The listing builds one solid part. Answer for the finished solid, in the listing's coordinates (mm). Face numbers are marked on the shaded views. A direction names the side the tool comes from. Give positions to 0.01 mm unless a question says otherwise; leave off trailing zeros. Write each loop counter-clockwise with the first axis right and the second up, starting at its lowest first coordinate (ties: lowest second). Pieces come first, ordered by that corner, then holes. Notation, with made-up numbers: M 34.25,2.25 L 89.25,2.25 A21 ccw 89.25,37.25 Z; hole C 57,-31 d10. An arc over 180 degrees is marked long. Return JSON: item names as keys, results as strings.
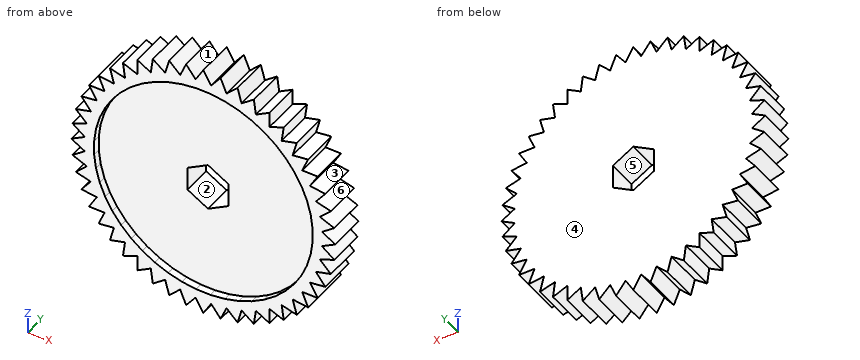
from build123d import *

# Parameters (mm, degrees)
SKETCH1_R           = 19.05
BOSS_EXTRUDE1_DEPTH = 5.08
BOSS_EXTRUDE3_DEPTH = 6.35
CIRPATTERN1_COUNT   = 48
CUT_EXTRUDE1_DEPTH  = 33.725610766


with BuildPart() as part:
    # Sketch1 → Boss-Extrude1 (new body)
    with BuildSketch(Plane(origin=(0, 0, 0), x_dir=(1, 0, 0), z_dir=(0, 1, 0))):
        with Locations(Location((0, 0, 0), (0, 0, 270))):
            Circle(SKETCH1_R)
    extrude(amount=BOSS_EXTRUDE1_DEPTH)

    # Sketch3 → Boss-Extrude3 (add)
    with BuildSketch(Plane(origin=(0, 5.08, 0), x_dir=(1, 0, 0), z_dir=(0, 1, 0))):
        Polygon((0, 22.86), (2.278670365, 18.913227154), (-2.278670365, 18.913227154), align=None)
    boss_extrude3 = extrude(amount=-BOSS_EXTRUDE3_DEPTH)

    # CirPattern1: Boss-Extrude3 ×48 about axis
    cirpattern1_axis = Axis((0, 0, 0), (0, 1, 0))
    for i in range(1, CIRPATTERN1_COUNT):
        add(boss_extrude3.rotate(cirpattern1_axis, i * 360 / CIRPATTERN1_COUNT))

    # Sketch6 → Cut-Extrude1 (cut, through all)
    with BuildSketch(Plane.XZ):
        Polygon((0, -4.106115114), (3.556, -2.053057557), (3.556, 2.053057557), (0, 4.106115114), (-3.556, 2.053057557), (-3.556, -2.053057557), align=None)
    extrude(amount=-CUT_EXTRUDE1_DEPTH, mode=Mode.SUBTRACT)


solid = part.part
Item 1: Which of the six approach directions +Z, -Z, +X, -X, +Y, -Y give full straight-line access (tool end or side, diameter ignored) to the marked faces 1, 2 and 3?
Geometry results:
{"face 1": "+Z, +Y, -Y", "face 2": "+Y, -Y", "face 3": "+X, +Y, -Y"}
Item 2: A cutting plane is placed at A-A, the plane z = -5. Write down the section's boundary in (x, y).
Geometry results:
{"outline": "M -21.16,-1.27 L -18.24,-1.27 L -18.24,0 L 18.24,0 L 18.24,-1.27 L 21.16,-1.27 L 21.16,5.08 L -21.16,5.08 Z"}
Item 3: A cutting plane is placed at B-B, the plane x = 10. Write down the section's boundary in (y, z).
Geometry results:
{"outline": "M -1.27,-18.97 L 5.08,-18.97 L 5.08,18.97 L -1.27,18.97 L -1.27,16.07 L 0,16.07 L 0,-16.07 L -1.27,-16.07 Z"}
Item 4: Determine the mould class of the marked faces 4, 5 and 6 for opening direction X: +X half, -X half, draft (parallel to the pull), parting line (faces both ways), or undercut.
Geometry results:
{"face 4": "draft", "face 5": "undercut", "face 6": "+X half"}
Item 5: Given pin 1 Ø3 at (y, z) = (3.5, -18) entering from +X; pin 2 Ø1.3 at (x, y) = (-18, 1.5) entering from -Z; pin 3 Ø0.8 at (y, z) = (3, 18.5) entering from -X, each flat-ended and moving along its own axis, determine where each tip first touches the part or whether it passes through.
Geometry results:
{"pin 1": "stops at x = 13.92", "pin 2": "stops at z = -13.92", "pin 3": "stops at x = -13.92"}
Item 6: Find the intervals of material crossed by line 1 (Z direction, x = -17.5, y = 1); line 2 (Z direction, x = 21.5, y = 1.25); line 3 (Z direction, x = 2, y = -0.5), in increasing order.
Geometry results:
{"line 1": "z = -13.83 to -12.38, -11.43 to 11.43, 12.38 to 13.83", "line 2": "z = -6.07 to -5.34, -3.47 to -2.09, -0.79 to 0.79, 2.09 to 3.47, 5.34 to 6.07", "line 3": "z = -21.38 to -18.81, 18.81 to 21.38"}
